Could you check a few things on this drawing? It's one solid part, dimensions in mm from its lowest x, y, z. A direction names the side the tool comes from. Coordinates: 2 decimals unless noted, no trailing zeros. Write each loop counter-clockwise with the first axis right and the second up, starting at its lowest first coordinate (ties: lowest second). Pieces come first, ordered by that corner, then holes.
Item 1: For the marked faces 1, 2 and 3, which set-ups out of +Z, -Z, +X, -X, +Y, -Y let a thin tool reach every point of the face, with its end or its side?
Item 2: If we mould it in two halves opening along Y, with no side actions, what happens to the marked faces 4, 5 and 6? For each: pulls with the +Y half, pulls with the -Y half, needs draft (parallel to the pull), parting line crosses it, or undercut.
Item 3: I want a section at B-B (y = 61). Please give me the cut outline in (x, z), and give its area (3 significant figures).
Item 4: Please list where these lines run through material, in increasing order: line 1 (Y direction, x = 31.5, z = 10) (1 decimal); line 2 (Y direction, x = 25, z = 10.5) (1 decimal); line 3 (Z direction, x = 34, y = 52).
Item 5: I want a section at A-A (z = 3). Please give me the cut outline in (x, y).
Item 6: I want a section at C-C (z = 27). Please give me the cut outline in (x, y), and give its area (3 significant figures).
Item 7: I'm going to push flat-ended pins straight in: P1, Ø24, axis at x = 26, y = 61, coming from the +Z side; P2, Ø3, axis at y = 63.5, z = 7, coming from the -X side; P3, Ø2, axis at x = 11.5, z = 26.5, coming from the +Y side; P4, Ø12.5, axis at x = 26.21, y = 61, coming from the +Z side. Where does each tip first touch, or does it pass through?
Item 8: I want a section at D-D (x = 38.5). Please give me the cut outline in (y, z).
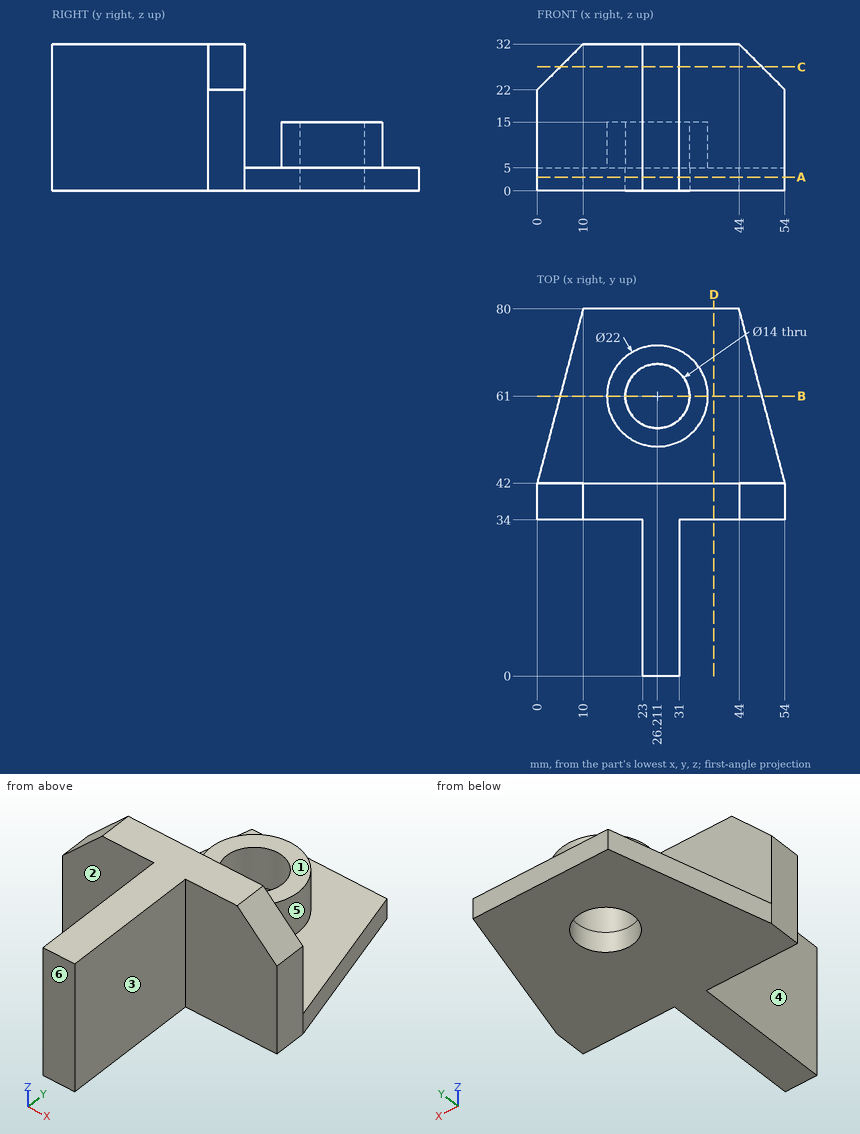
Answer:
1. face 1: +Z, +X, -X, +Y
1. face 2: +Z, -Z, -X, -Y
1. face 3: +Z, -Z, +X, -Y
2. face 4: needs draft
2. face 5: undercut
2. face 6: pulls with the -Y half
3. outline: (5, 0) - (19.21, 0) - (19.21, 15) - (15.21, 15) - (15.21, 5) - (5, 5) - close; (33.21, 0) - (49, 0) - (49, 5) - (37.21, 5) - (37.21, 15) - (33.21, 15) - close
3. area: 230 mm2
4. line 1: y = 34 to 42, 51.4 to 56.4, 65.6 to 70.6
4. line 2: y = 0 to 42, 50.1 to 54.1, 67.9 to 71.9
4. line 3: z = 0 to 5
5. outline: (0, 34) - (23, 34) - (23, 0) - (31, 0) - (31, 34) - (54, 34) - (54, 42) - (44, 80) - (10, 80) - (0, 42) - close; hole circle Ø14 at (26.21, 61)
6. outline: (5, 34) - (23, 34) - (23, 0) - (31, 0) - (31, 34) - (49, 34) - (49, 42) - (5, 42) - close
6. area: 624 mm2
7. P1: stops at z = 15
7. P2: stops at x = 15.26
7. P3: stops at y = 42
7. P4: passes through
8. outline: (34, 0) - (80, 0) - (80, 5) - (42, 5) - (42, 32) - (34, 32) - close
